Check sheet for the modelled part. Datum: model origin and axes. Units: mm. Face numbers are marked on the shaded views. A direction names the side the tool comes from. Give positions to 0.01 mm unless a question says otherwise; leave off trailing zeros. Write each loop counter-clockwise with the first axis right and the second up, starting at its lowest first coordinate (ties: lowest second). Pieces come first, ordered by that corner, then holes. Notation, with made-up numbers: M -27,86.25 L 25,86.25 A11 ccw 25,90.25 Z; hole C 13,-12.75 d3. An arc over 180 degrees is marked long. One line per item, written item: value. Start each with the question number.
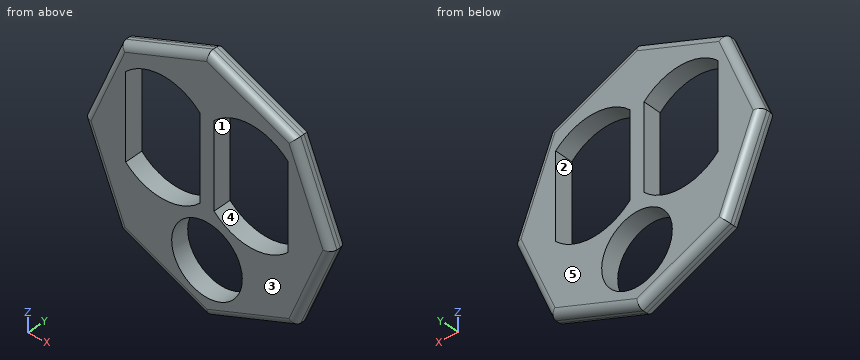
from build123d import *

# Parameters (mm, degrees)
BOSS_EXTRUDE1_DEPTH = 5
SKETCH4_W           = 21
SKETCH4_H           = 24
CUT_EXTRUDE1_DEPTH  = 5
CUT_EXTRUDE2_DEPTH  = 5
SKETCH10_W          = 47.253020793
SKETCH10_H          = 79.148030785
CUT_EXTRUDE3_DEPTH  = 5
MIRROR8_DEPTH       = 5
SKETCH11_R          = 10
CUT_EXTRUDE4_DEPTH  = 5
FILLET5_R           = 2


# Read off the part's stored shape, not the designer's step: Mirror8
with BuildPart() as part:
    # Sketch3 → Boss-Extrude1 (new body)
    with BuildSketch(Plane(origin=(0, 0, 0), x_dir=(1, 0, 0), z_dir=(0, 1, 0))):
        Polygon((35, 0), (24.748737342, 24.748737342), (0, 35), (-24.748737342, 24.748737342), (-35, 0), (-24.748737342, -24.748737342), (0, -35), (24.748737342, -24.748737342), align=None)
    extrude(amount=BOSS_EXTRUDE1_DEPTH)

    # Sketch4 → Cut-Extrude1 (cut)
    with BuildSketch(Plane(origin=(0, 5, 0), x_dir=(1, 0, 0), z_dir=(0, 1, 0))):
        with Locations((-12.508622631, -6.229175633)):
            Rectangle(SKETCH4_W, SKETCH4_H)
    extrude(amount=-CUT_EXTRUDE1_DEPTH, mode=Mode.SUBTRACT)

    # Sketch4<6> → Cut-Extrude2 (cut)
    with BuildSketch(Plane(origin=(0, 5, 0), x_dir=(1, 0, 0), z_dir=(0, 1, 0))):
        with BuildLine():
            ThreePointArc((-23.008622631, 5.770824367), (-12.508622631, 10.120066772), (-2.008622631, 5.770824367))
            Line((-2.008622631, 5.770824367), (-23.008622631, 5.770824367))
        make_face()
        with BuildLine():
            Line((-23.008622631, -18.229175633), (-2.008622631, -18.229175633))
            ThreePointArc((-2.008622631, -18.229175633), (-12.508622631, -22.578418038), (-23.008622631, -18.229175633))
        make_face()
    extrude(amount=-CUT_EXTRUDE2_DEPTH, mode=Mode.SUBTRACT)

    # Sketch10 → Cut-Extrude3 (cut)
    with BuildSketch(Plane(origin=(0, 5, 0), x_dir=(1, 0, 0), z_dir=(0, 1, 0))):
        with Locations((23.626510397, -1.493894903)):
            Rectangle(SKETCH10_W, SKETCH10_H)
    extrude(amount=-CUT_EXTRUDE3_DEPTH, mode=Mode.SUBTRACT)

    # Mirror8 outline → Mirror8 (add)
    with BuildSketch(Plane(origin=(0, 0, 0), x_dir=(1, 0, 0), z_dir=(0, 1, 0))):
        Polygon((24.748737342, 24.748737342), (0, 35), (0, -35), (24.748737342, -24.748737342), (35, 0), align=None)
        with BuildLine():
            ThreePointArc((2.008622631, 5.770824367), (12.508622631, 10.120066772), (23.008622631, 5.770824367))
            Line((23.008622631, 5.770824367), (23.008622631, -18.229175633))
            ThreePointArc((23.008622631, -18.229175633), (12.508622631, -22.578418038), (2.008622631, -18.229175633))
            Line((2.008622631, -18.229175633), (2.008622631, 5.770824367))
        make_face(mode=Mode.SUBTRACT)
    extrude(amount=MIRROR8_DEPTH)

    # Sketch11 → Cut-Extrude4 (cut)
    with BuildSketch(Plane(origin=(0, 5, 0), x_dir=(1, 0, 0), z_dir=(0, 1, 0))):
        with Locations(Location((0, 19.772592196, 0), (0, 0, 270))):
            Circle(SKETCH11_R)
    extrude(amount=-CUT_EXTRUDE4_DEPTH, mode=Mode.SUBTRACT)

    # Fillet5
    fillet5_edges = [part.edges().sort_by_distance(p)[0] for p in [
        (-12.374368671, 5, -29.874368671),
        (-29.874368671, 5, -12.374368671),
        (-29.874368671, 5, 12.374368671),
        (-12.374368671, 5, 29.874368671),
        (12.374368671, 5, -29.874368671),
        (29.874368671, 5, -12.374368671),
        (29.874368671, 5, 12.374368671),
        (12.374368671, 0, -29.874368671),
        (29.874368671, 0, -12.374368671),
        (29.874368671, 0, 12.374368671),
        (12.374368671, 0, 29.874368671),
        (12.374368671, 5, 29.874368671),
        (-12.374368671, 0, 29.874368671),
        (-29.874368671, 0, 12.374368671),
        (-29.874368671, 0, -12.374368671),
        (-12.374368671, 0, -29.874368671),
    ]]
    fillet(fillet5_edges, radius=FILLET5_R)


solid = part.part
1) Draft check along X on the marked faces 1, 2 and 3. Enter one of: released by +X, released by -X, zero draft, split by the parting line, or undercut.
2) Cross-section at B-B (x = -6). State how many separate pieces and enclosed holes the cut face has, plus the area to 3 significant figures.
3) Gauge pin test, flat ends, axial feed: pin 1 (1.5 mm diameter, centred on x = 4, y = 3.5, fed in from -Z); pin 2 (1.5 mm diameter, centred on y = 2.5, z = 4, fed in from -X); pin 3 (2.5 mm diameter, centred on y = 3, z = 5.5, fed in from +X); pin 4 (18 mm diameter, centred on x = 0, z = -19.77, fed in from -Y). Record the tip position at first contact, or that the pin passes through.
4) Material ranges on L1, parallel to X at y = 0.55, z = 21; L2, parallel to X at y = 0.55, z = -9; L3, parallel to Z at x = -3.5, y = 1.6, recorded low to high. Write a range as from..to.
5) Cross-section at A-A (y = 3.85). Record the boundary of the cut face in (x, z).
6) Tool access check on the marked faces 4 and 5. Record the directions out of +Z, -Z, +X, -X, +Y, -Y that give a thin tool (end or side, any length) a straight path to the whole face; none if there is none.
Data:
1. face 1: undercut
1. face 2: undercut
1. face 3: zero draft
2. separate pieces: 3
2. enclosed holes: 0
2. area: 93.0 mm2
3. pin 1: stops at z = -33.62
3. pin 2: stops at x = -33.65
3. pin 3: stops at x = 33.24
3. pin 4: passes through
4. L1: x = -25.63..-19.17, -5.85..5.85, 19.17..25.63
4. L2: x = -30.6..-18.17, -6.85..6.85, 18.17..30.6
4. L3: z = -33.51..-29.14, -10.41..-7.08, 19.53..33.51
5. outline: M -34.79,0 L -24.6,-24.6 L 0,-34.79 L 24.6,-24.6 L 34.79,0 L 24.6,24.6 L 0,34.79 L -24.6,24.6 Z; hole M -23.01,-5.77 A14.85 ccw -2.01,-5.77 L -2.01,18.23 A14.85 ccw -23.01,18.23 Z; hole C 0,-19.77 d20; hole M 2.01,-5.77 A14.85 ccw 23.01,-5.77 L 23.01,18.23 A14.85 ccw 2.01,18.23 Z
6. face 4: +Y, -Y
6. face 5: +Z, -Z, +X, -X, +Y
